Verification items for this drawing (mm, ordinates from the low corner). Give positions to 0.01 mm unless a question says otherwise; leave off trailing zeros. Write each loop counter-clockwise with the first axis right and the second up, starting at its lowest first coordinate (ties: lowest second). Pieces come first, ordered by that corner, then holes. Notation, with made-up numbers: M 48,-30.75 L 60,-30.75 A19 ccw 60,0.25 Z; hole C -33.75,64 d2. An arc over 180 degrees is marked long. Write each question's results on one line, items separated by ' | '.
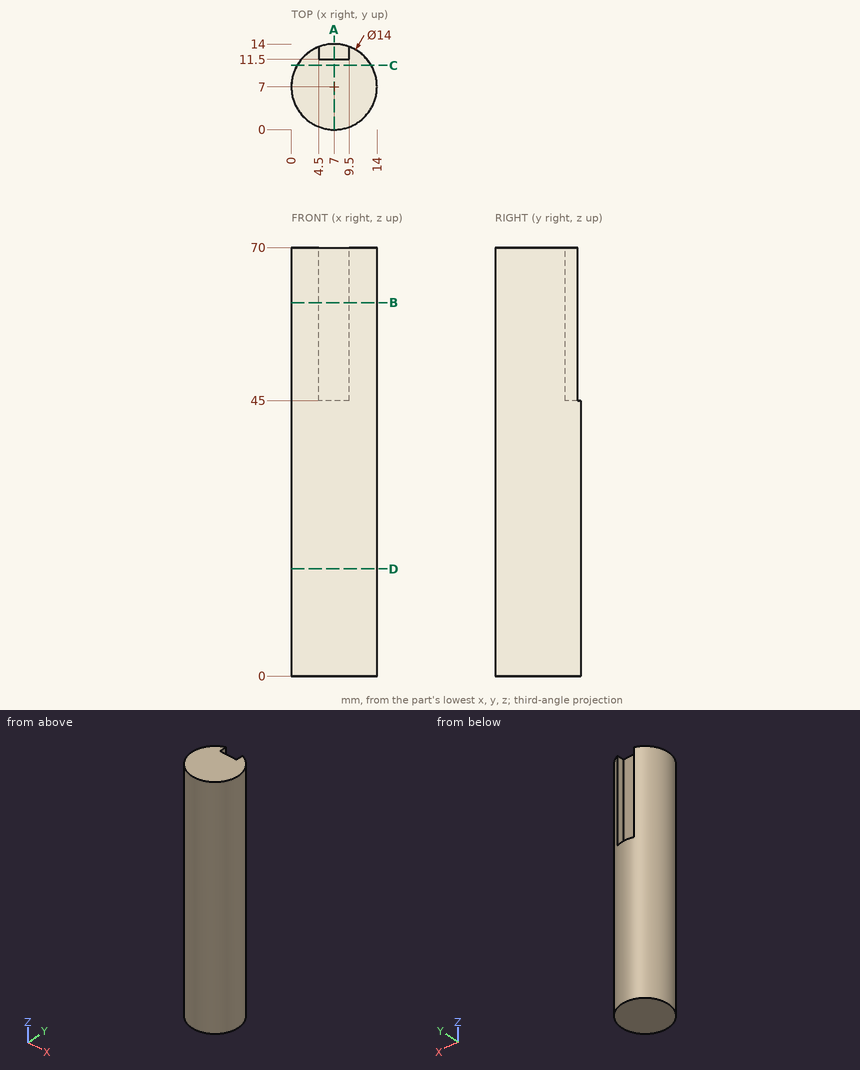
Q1. Section check A-A (x = 7). Enter the section's corners in (y, z).
Answer key:
outline: M 0,0 L 14,0 L 14,45 L 11.5,45 L 11.5,70 L 0,70 Z
Q2. Material ranges on probe 1 along Z at (x, y) = (8, 13); probe 2 along Y at (x, z) = (7.25, 9); probe 3 along X at (y, z) = (8, 13.5), recorded low to high. Write a range as [from, to].
Answer key:
probe 1: z = [0, 45] | probe 2: y = [0, 14] | probe 3: x = [0.07, 13.93]
Q3. Section check D-D (z = 17.5). Enter the section's corners in (x, y).
Answer key:
outline: C 7,7 d14
Q4. Section check B-B (z = 61). Enter the section's corners in (x, y).
Answer key:
outline: M 4.5,11.5 L 4.5,13.54 A7 ccw long 9.5,13.54 L 9.5,11.5 Z
Q5. Section check C-C (y = 10.5). Enter the section's corners in (x, z), then the cut area to 3 significant figures.
Answer key:
outline: M 0.94,0 L 13.06,0 L 13.06,70 L 0.94,70 Z | area: 849 mm2
Q6. Depth check by flat-ended pin: P1, Ø3, axis at x = 10, z = 19.5, coming from the -Y side; P2, Ø5.5, axis at x = 6, z = 62.5, coming from the +Y side; P3, Ø2, axis at y = 12.5, z = 60, coming from the +X side. Enter the tip coordinate at first touch or a pass-through.
Answer key:
P1: stops at y = 0.16 | P2: stops at y = 13.54 | P3: stops at x = 12.36
